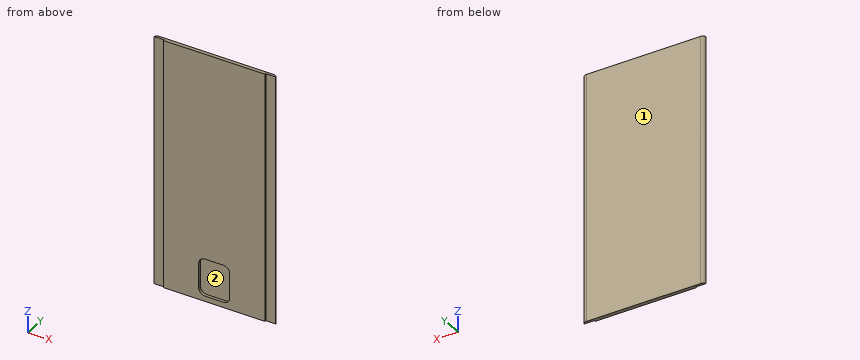
from build123d import *

# Parameters (mm, degrees)
SKIZZE2_W                       = 98
SKIZZE2_H                       = 200
AUFSATZ_LINEAR_AUSTRAGEN2_DEPTH = 1.5
SKIZZE4_W                       = 8
SKIZZE4_H                       = 200
SCHNITT_LINEAR_AUSTRAGEN1_DEPTH = 1
VERRUNDUNG1_R                   = 3
SKIZZE5_W                       = 25
SKIZZE5_H                       = 30
SCHNITT_LINEAR_AUSTRAGEN2_DEPTH = 2.5
VERRUNDUNG2_R                   = 5


with BuildPart() as part:
    # Skizze2 → Aufsatz-Linear austragen2 (new, symmetric)
    with BuildSketch(Plane(origin=(0, 0, 0), x_dir=(1, 0, 0), z_dir=(0, 1, 0))):
        Rectangle(SKIZZE2_W, SKIZZE2_H)
    extrude(amount=AUFSATZ_LINEAR_AUSTRAGEN2_DEPTH, both=True)

    # Skizze4 → Schnitt-Linear austragen1 (cut)
    with BuildSketch(Plane.XZ.offset(1.5)):
        with Locations((-45, 0)):
            Rectangle(SKIZZE4_W, SKIZZE4_H)
        with Locations((45, 0)):
            Rectangle(SKIZZE4_W, SKIZZE4_H)
    extrude(amount=-SCHNITT_LINEAR_AUSTRAGEN1_DEPTH, mode=Mode.SUBTRACT)

    # Verrundung1
    # the kernel refuses this fillet: 3 mm, written as the material it takes off along each edge
    with BuildSketch(Plane(origin=(-49, 1.5, 107.071067812), x_dir=(0, -1, 0), z_dir=(0, 0, -1))) as verrundung1_piece_1:
        with BuildLine():
            CenterArc((3, -2.828427125), VERRUNDUNG1_R, 109.471220634, 70.528779366)
            Line((0, -2.828427125), (-0.06, -2.828427125))
            Line((-0.06, -2.828427125), (-0.06, 0))
            Line((-0.06, 0), (0, 0.06))
            ThreePointArc((0, 0.06), (1, 0.06), (1.98, 0.056568542))
            Line((1.98, 0.056568542), (2, 0))
        make_face()
    extrude(amount=214.142135624, mode=Mode.SUBTRACT)
    with BuildSketch(Plane(origin=(49, 1.5, -107.071067812), x_dir=(-1, 0, 0), z_dir=(0, 0, 1))) as verrundung1_piece_2:
        with BuildLine():
            CenterArc((2.828427125, 3), VERRUNDUNG1_R, 199.471220634, 70.528779366)
            Line((0, 2), (-0.056568542, 1.98))
            ThreePointArc((-0.056568542, 1.98), (-0.06, 1), (-0.06, 0))
            Line((-0.06, 0), (0, -0.06))
            Line((0, -0.06), (2.828427125, -0.06))
            Line((2.828427125, -0.06), (2.828427125, 0))
        make_face()
    extrude(amount=214.142135624, mode=Mode.SUBTRACT)

    # Skizze5 → Schnitt-Linear austragen2 (cut)
    with BuildSketch(Plane.XZ.offset(1.5)):
        with Locations((0, -80.75)):
            Rectangle(SKIZZE5_W, SKIZZE5_H)
    extrude(amount=-SCHNITT_LINEAR_AUSTRAGEN2_DEPTH, mode=Mode.SUBTRACT)

    # Verrundung2
    verrundung2_edges = [part.edges().sort_by_distance(p)[0] for p in [
        (-12.5, -0.25, -95.75),
        (-12.5, -0.25, -65.75),
        (12.5, -0.25, -65.75),
        (12.5, -0.25, -95.75),
    ]]
    fillet(verrundung2_edges, radius=VERRUNDUNG2_R)


solid = part.part
CAD build for the part. Positions are in the model's coordinates, mm. Face numbers are marked on the shaded views. Coordinates: 2 decimals unless noted, no trailing zeros. Loops run counter-clockwise (first coordinate to the right, second up) from the corner with the lowest first, then second, coordinate; pieces in that order, holes last. Notation, with made-up numbers: (-16, 54.5) - (32, 54.5) arc R28 ccw to (32, 73.5) - close; hole circle Ø5 at (37.5, -25). An arc over 180 degrees is marked (long way). Use one line per item in the form item = value. Start each with the question number.
1) Band-saw the part on C-C (x = 2.5). Give the cut face in (y, z).
2) Drill centre lines: L1, parallel to X at y = -0.65, z = -86; L2, parallel to Z at x = 4.5, y = 0.55; L3, parallel to Y at x = -44, z = 48.5. Where is each one in solid material? Low to high. Write a range as from..to.
3) Band-saw the part on B-B (y = 0.1). Give the cut face in (x, z), and give its area (3 significant figures).
4) Flat gauge pins, fed straight in: pin 1 (0.5 mm diameter, centred on y = -1, z = -34.5, fed in from +X); pin 2 (2.5 mm diameter, centred on x = -46, z = 3.5, fed in from -Y); pin 3 (1.1 mm diameter, centred on y = -1, z = 31.5, fed in from -X); pin 4 (7.5 mm diameter, centred on x = -3, z = -76, fed in from -Y). Where does each tip first touch, or does it go through?
5) Two-plate mould, pull along X, no slides. Class the marked faces 1 and 2: +X half, -X half, draft (parallel to the pull), parting line (faces both ways), or undercut.
6) Band-saw the part on A-A (z = -32.5). Give the cut face in (x, y).
Check values:
q1.outline = (-1.5, -100) - (1.5, -100) - (1.5, 100) - (-1.5, 100) - (-1.5, -65.75) - (1, -65.75) - (1, -95.75) - (-1.5, -95.75) - close
q2.L1 = -41..-12.5, 12.5..41
q2.L2 = -100..-95.75, -65.75..100
q2.L3 = -0.5..1.5
q3.outline = (-48.71, -100) - (48.71, -100) - (48.71, 100) - (-48.71, 100) - close; hole (-12.5, -90.75) arc R5 ccw to (-7.5, -95.75) - (7.5, -95.75) arc R5 ccw to (12.5, -90.75) - (12.5, -70.75) arc R5 ccw to (7.5, -65.75) - (-7.5, -65.75) arc R5 ccw to (-12.5, -70.75) - close
q3.area = 18,800 mm2
q4.pin_1 = 41
q4.pin_2 = -0.5
q4.pin_3 = -49
q4.pin_4 = 1
q5.face_1 = draft
q5.face_2 = undercut
q6.outline = (-49, -0.5) - (-41, -0.5) - (-41, -1.5) - (41, -1.5) - (41, -0.5) - (49, -0.5) arc R3 ccw to (46.17, 1.5) - (-46.17, 1.5) arc R3 ccw to start
